Verification items for the finished model (mm, model axes). A direction names the side the tool comes from. Round coordinates to 2 decimals unless told otherwise and drop trailing zeros. Write each loop counter-clockwise with the first axis right and the second up, starting at its lowest first coordinate (ties: lowest second). Pieces come first, ordered by that corner, then holes. Notation, with made-up numbers: M 36,79 L 90,79 A3 cw 90,83 Z; hole C -13.5,23.25 d8. An arc over 180 degrees is marked long. One line per question, with ' | ' between items.
from build123d import *

# Parameters (mm, degrees)
BOSS_EXTRUDE1_DEPTH = 1.5
SKETCH2_W           = 2.713539356
SKETCH2_H           = 31.847242959
BOSS_EXTRUDE2_DEPTH = 2
CUT_EXTRUDE1_DEPTH  = 0.75
FILLET1_R           = 1
FILLET2_R           = 0.3
CUT_EXTRUDE2_DEPTH  = 1.2


with BuildPart() as part:
    # Sketch1 → Boss-Extrude1 (new body)
    with BuildSketch(Plane.XY):
        Polygon((13.150722075, -0.506964629), (13.150722075, -7.292554302), (20.475117676, -7.292554302), (20.475117676, 24.554688657), (13.150722075, 24.554688657), (13.150722075, 17.625640453), (-2.779550764, 17.625640453), (-2.779550764, 15.652441277), (-4.09999988, 15.652441277), (-4.09999988, 1.623886225), (-2.779550764, 1.623886225), (-2.779550764, -0.506964629), align=None)
    extrude(amount=-BOSS_EXTRUDE1_DEPTH)

    # Sketch2 → Boss-Extrude2 (add)
    with BuildSketch(Plane(origin=(0, 0, -1.5), x_dir=(-1, 0, 0), z_dir=(0, 0, -1))):
        with Locations((-19.118347998, 8.631067178)):
            Rectangle(SKETCH2_W, SKETCH2_H)
    extrude(amount=BOSS_EXTRUDE2_DEPTH)

    # Sketch3 → Cut-Extrude1 (cut)
    with BuildSketch(Plane(origin=(0, 0, -1.5), x_dir=(-1, 0, 0), z_dir=(0, 0, -1))):
        Polygon((2.779550764, 15.589201664), (-9.466641169, 15.589201664), (-9.466641169, 1.649000414), (2.779550764, 1.649000414), (2.779550764, 1.623886225), (4.09999988, 1.623886225), (4.09999988, 15.589201664), align=None)
    extrude(amount=-CUT_EXTRUDE1_DEPTH, mode=Mode.SUBTRACT)

    # Fillet1
    fillet1_edges = [part.edges().sort_by_distance(p)[0] for p in [
        (17.76157832, 8.631067178, -1.5),
    ]]
    fillet(fillet1_edges, radius=FILLET1_R)

    # Fillet2
    fillet2_edges = [part.edges().sort_by_distance(p)[0] for p in [
        (3.343545202, 1.649000414, -1.5),
        (9.466641169, 8.619101039, -1.5),
        (2.683320645, 15.589201664, -1.5),
    ]]
    fillet(fillet2_edges, radius=FILLET2_R)

    # Sketch4 → Cut-Extrude2 (cut)
    with BuildSketch(Plane(origin=(20.475117676, 0, 0), x_dir=(0, 0, -1), z_dir=(1, 0, 0))):
        with BuildLine():
            Line((1.679428172, 22.66130131), (1.679429396, -5.33869869))
            ThreePointArc((1.679429396, -5.33869869), (2.265215896, -6.752912227), (3.679429484, -7.338698602))
            Line((3.679429484, -7.338698602), (3.679428085, 24.661301398))
            ThreePointArc((3.679428085, 24.661301398), (2.265214548, 24.075514898), (1.679428172, 22.66130131))
        make_face()
    extrude(amount=-CUT_EXTRUDE2_DEPTH, mode=Mode.SUBTRACT)


solid = part.part
1. Go/stop test with flat-tipped pins: P1, Ø8, axis at x = 9.5, y = 17.5, coming from the +Z side; P2, Ø1.5, axis at x = -3, z = -1, coming from the +Y side; P3, Ø0.6, axis at x = 20, y = 7, coming from the -Z side; P4, Ø10, axis at x = 4.5, y = 6, coming from the -Z side. Record where each tip stops, or that it passes through.
Results:
P1: stops at z = 0 | P2: stops at y = 17.63 | P3: stops at z = -1.68 | P4: stops at z = -1.5
2. Section check C-C, the plane y = 6. Record the cut outline in (x, z), then the cut area to 3 significant figures.
Results:
outline: M -4.1,-0.75 L 9.47,-0.75 L 9.47,-1.2 A0.3 ccw 9.77,-1.5 L 16.76,-1.5 A1 cw 17.76,-2.5 L 17.76,-3.5 L 19.28,-3.5 L 19.28,-1.68 L 20.48,-1.68 L 20.48,0 L -4.1,0 Z | area: 30.1 mm2
3. Section check B-B, the plane y = 17. Record the cut outline in (x, z), then the cut area to 3 significant figures.
Results:
outline: M -2.78,-1.5 L 16.76,-1.5 A1 cw 17.76,-2.5 L 17.76,-3.5 L 19.28,-3.5 L 19.28,-1.68 L 20.48,-1.68 L 20.48,0 L -2.78,0 Z | area: 38.3 mm2
4. Section check D-D, the plane x = 16.25. Record the cut outline in (y, z).
Results:
outline: M -7.29,-1.5 L 24.55,-1.5 L 24.55,0 L -7.29,0 Z
5. Thickness scan on line 1 (Z direction, x = 14.75, y = 13.5); line 2 (Y direction, x = -1.75, z = -0.3); line 3 (Z direction, x = 3.25, y = 14). Record the ranges inside material, lowest first.
Results:
line 1: z = -1.5 to 0 | line 2: y = -0.51 to 17.63 | line 3: z = -0.75 to 0
6. Section check A-A, the plane x = 4.25. Record the cut outline in (y, z).
Results:
outline: M -0.51,-1.5 L 1.35,-1.5 A0.3 ccw 1.65,-1.2 L 1.65,-0.75 L 15.59,-0.75 L 15.59,-1.2 A0.3 ccw 15.89,-1.5 L 17.63,-1.5 L 17.63,0 L -0.51,0 Z
7. Tool access check on faces 1 (the face through (5, 17.626, -1)), 2 (the face through (3, 9, -0.75)), 3 (the face through (19.88, -6.58, -2.11)), 4 (the face through (17.762, 8, -3)). Record the directions out of +Z, -Z, +X, -X, +Y, -Y that give a thin tool (end or side, any length) a straight path to the whole face; none if there is none.
Results:
face 1: +Z, -Z, -X, +Y | face 2: -Z, -X | face 3: -Z, +X | face 4: -Z, -X, +Y, -Y
